Here's the drawing with two shaded views (mm, measured from the low corner). I have some questions. Give positions to 0.01 mm unless a question says otherwise; leave off trailing zeros. Loops run counter-clockwise (first coordinate to the right, second up) from the corner with the lowest first, then second, coordinate; pieces in that order, holes last. Notation, with made-up numbers: M -20,-17 L -12,-17 A23 ccw -12,-8 Z; hole C 1.25,47 d9. An arc over 180 degrees is marked long. Put each result on its own line as item: value. Start each with the question number.
1) Imagine slicing it at A-A (z = 15.95). Write out the boundary of the cut face in (x, y).
2) Please list where these lines run through material, in increasing order: line 1 along Z through (x, y) = (22.5, 0.7); line 2 along X through (y, z) = (2.9, 15.95); line 3 along X through (y, z) = (1.35, 56.55). Write a range as from..to.
3) Imagine slicing it at D-D (z = 56). Write out the boundary of the cut face in (x, y), then the cut area to 3 significant figures.
4) For P1, Ø2.5, axis at x = 36.5, y = 2.5, coming from the -Z side; P2, Ø1.5, axis at y = 1.5, z = 69, coming from the +X side; P3, Ø1.5, axis at y = 3, z = 3, coming from the -X side; P4, Ø2, axis at x = 22.5, z = 15.95, coming from the -Y side, each with a flat end and sliding along its axis, tell me the tip position at first contact or that it passes through.
5) Imagine slicing it at B-B (x = 22.5). Write out the boundary of the cut face in (y, z), then the cut area to 4 significant figures.
6) Imagine slicing it at C-C (y = 0.75). Write out the boundary of the cut face in (x, z).
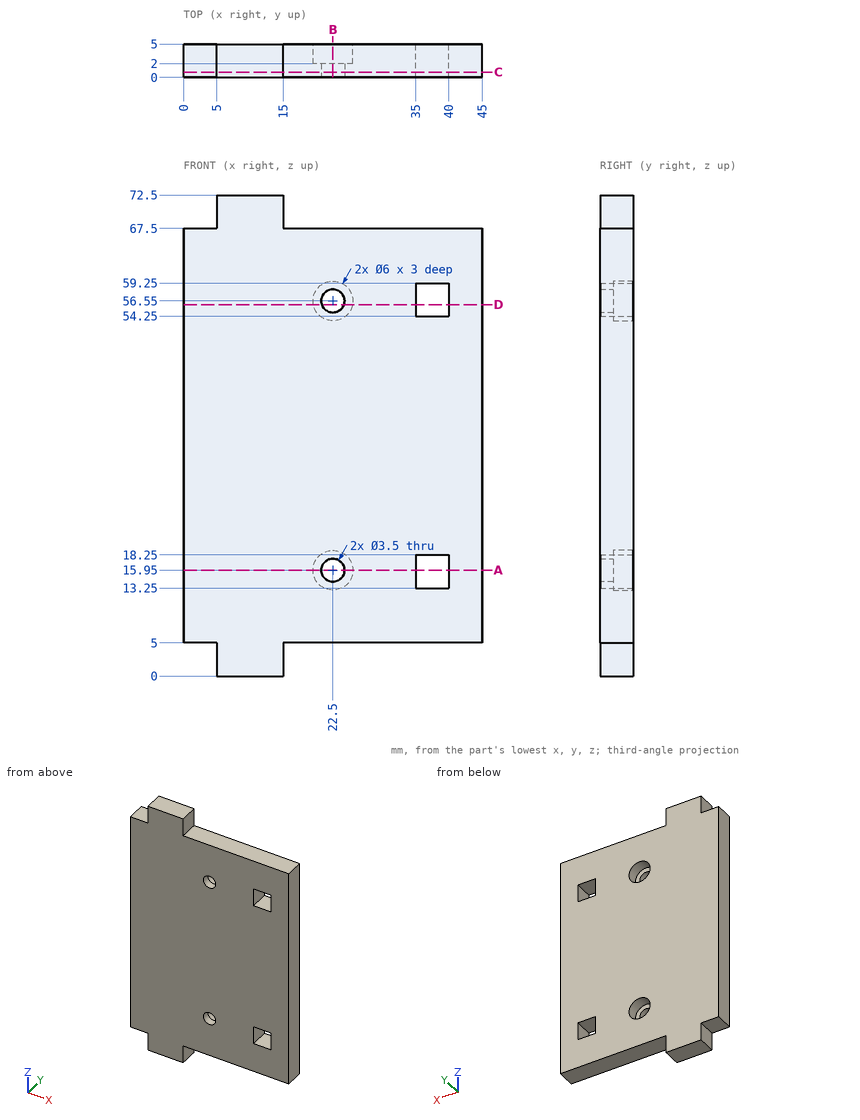
Recorded:
1. outline: M 0,0 L 20.75,0 L 20.75,2 L 19.5,2 L 19.5,5 L 0,5 Z; M 24.25,0 L 35,0 L 35,5 L 25.5,5 L 25.5,2 L 24.25,2 Z; M 40,0 L 45,0 L 45,5 L 40,5 Z
2. line 1: 5..14.2, 17.7..54.8, 58.3..67.5
2. line 2: 0..19.5, 25.5..35, 40..45
2. line 3: 0..20.75, 24.25..35, 40..45
3. outline: M 0,0 L 20.84,0 L 20.84,2 L 19.55,2 L 19.55,5 L 0,5 Z; M 24.16,0 L 35,0 L 35,5 L 25.45,5 L 25.45,2 L 24.16,2 Z; M 40,0 L 45,0 L 45,5 L 40,5 Z
3. area: 176 mm²
4. P1: z = 5
4. P2: x = 15
4. P3: x = 5
4. P4: through
5. outline: M 0,5 L 5,5 L 5,12.95 L 2,12.95 L 2,14.2 L 0,14.2 Z; M 0,17.7 L 2,17.7 L 2,18.95 L 5,18.95 L 5,53.55 L 2,53.55 L 2,54.8 L 0,54.8 Z; M 0,58.3 L 2,58.3 L 2,59.55 L 5,59.55 L 5,67.5 L 0,67.5 Z
5. area: 262.5 mm²
6. outline: M 0,5 L 5,5 L 5,0 L 15,0 L 15,5 L 45,5 L 45,67.5 L 15,67.5 L 15,72.5 L 5,72.5 L 5,67.5 L 0,67.5 Z; hole C 22.5,15.95 d3.5; hole C 22.5,56.55 d3.5; hole M 35,13.25 L 40,13.25 L 40,18.25 L 35,18.25 Z; hole M 35,54.25 L 40,54.25 L 40,59.25 L 35,59.25 Z
